from build123d import *

# Parameters (mm, degrees)
PAD_DEPTH       = 30
SKETCH004_R     = 9.7
POCKET_DEPTH    = 29
SKETCH005_R     = 9.7
POCKET001_DEPTH = 29
SKETCH006_R     = 1.5
POCKET002_DEPTH = 10
SKETCH007_R     = 1.5
POCKET003_DEPTH = 10
PAD001_DEPTH    = 10
SKETCH008_R     = 2.1
POCKET004_DEPTH = 7
SKETCH009_R     = 3.6
POCKET005_DEPTH = 2
FILLET_R        = 5


with BuildPart() as pocket003:
    # Sketch → Pad (new body, symmetric)
    with BuildSketch(Plane.XY):
        with BuildLine():
            ThreePointArc((-5.656854, 5.656854), (0, -8), (5.656854, 5.656854))
            Line((10.606602, 10.606602), (5.656854, 5.656854))
            ThreePointArc((0, -15), (13.858193, -5.740251), (10.606602, 10.606602))
            Line((-4.3e-05, -15), (0, -15))
            ThreePointArc((-15, -4.3e-05), (-10.606602, -10.606602), (-4.3e-05, -15))
            Line((-15, 0), (-15, -4.3e-05))
            ThreePointArc((-10.606602, 10.606602), (-13.858193, 5.740251), (-15, 0))
            Line((-5.656854, 5.656854), (-10.606602, 10.606602))
        make_face()
    extrude(amount=PAD_DEPTH, both=True)

    # Sketch004 → Pocket (cut)
    with BuildSketch(Plane.XY.offset(30)):
        Circle(SKETCH004_R)
    extrude(amount=-POCKET_DEPTH, mode=Mode.SUBTRACT)

    # Sketch005 → Pocket001 (cut)
    with BuildSketch(Plane(origin=(0, 0, -30), x_dir=(1, 0, 0), z_dir=(0, 0, -1))):
        Circle(SKETCH005_R)
    extrude(amount=-POCKET001_DEPTH, mode=Mode.SUBTRACT)

    # Sketch006 → Pocket002 (cut)
    with BuildSketch(Plane.XY.offset(30)):
        with Locations((-8, -8.944272)):
            Circle(SKETCH006_R)
    extrude(amount=-POCKET002_DEPTH, mode=Mode.SUBTRACT)

    # Sketch007 → Pocket003 (cut)
    with BuildSketch(Plane(origin=(0, 0, -30), x_dir=(1, 0, 0), z_dir=(0, 0, -1))):
        with Locations((-8, 8.944272)):
            Circle(SKETCH007_R)
    extrude(amount=-POCKET003_DEPTH, mode=Mode.SUBTRACT)


with BuildPart() as fusion:
    # Sketch003 → Pad001 (new body, symmetric)
    with BuildSketch(Plane.XY):
        with BuildLine():
            ThreePointArc((-13, 0), (0, -13), (13, 0))
            Line((13, 0), (13, -8))
            Line((13, -8), (25, -8))
            Line((25, -15), (25, -8))
            Line((-25, -15), (25, -15))
            Line((-25, -8), (-25, -15))
            Line((-13, -8), (-25, -8))
            Line((-13, 0), (-13, -8))
        make_face()
    extrude(amount=PAD001_DEPTH, both=True)

    # Sketch008 → Pocket004 (cut)
    with BuildSketch(Plane.XZ.offset(15)):
        with Locations((-19, 0)):
            Circle(SKETCH008_R)
        with Locations((19, 0)):
            Circle(SKETCH008_R)
    extrude(amount=-POCKET004_DEPTH, mode=Mode.SUBTRACT)

    # Sketch009 → Pocket005 (cut)
    with BuildSketch(Plane(origin=(0, -8, 0), x_dir=(-1, 0, 0), z_dir=(0, 1, 0))):
        with Locations((-19, 0)):
            Circle(SKETCH009_R)
        with Locations((19, 0)):
            Circle(SKETCH009_R)
    extrude(amount=-POCKET005_DEPTH, mode=Mode.SUBTRACT)

    # Fillet
    fillet_edges = [fusion.edges().sort_by_distance(p)[0] for p in [
        (25, -11.5, 10),
        (25, -11.5, -10),
        (-25, -11.5, 10),
        (-25, -11.5, -10),
    ]]
    fillet(fillet_edges, radius=FILLET_R)

    # Fusion: union Pocket003
    add(pocket003.part)


solid = fusion.part
Source: CAD feature listing. Evaluate the final solid. Frame: model axes, mm. A direction names the side the tool comes from. Give positions to 0.01 mm unless a question says otherwise; leave off trailing zeros. Write each loop counter-clockwise with the first axis right and the second up, starting at its lowest first coordinate (ties: lowest second). Pieces come first, ordered by that corner, then holes. Notation, with made-up numbers: (39.25, 30) - (91.25, 30) arc R24 ccw to (91.25, 45) - close; hole circle Ø4 at (-15, 33). An arc over 180 degrees is marked (long way). Write item = value, one per line. Start each with the question number.
Q1. Cut plane B-B, the plane y = 2. Return loops of the section in (x, z), then the cut area to 3 significant figures.
Q2. Material intervals for probe 1 along Z at (x, y) = (-19, -13.7); probe 2 along Z at (x, y) = (-19, -9); probe 3 along X at (y, z) = (-7.25, 22.5), sorted ascending.
Q3. Reachability of faces 1 (the cylindrical face through (-13.663, -6.189, 0.42)), 2 (the flat face through (15, -12, -10)), 3 (the cylindrical face through (-15.403, -8.986, 0.158)) from +Z, -Z, +X, -X, +Y, -Y: full face, straight path, thin tool, end or side. Return the list, or none.
Q4. Cut plane A-A, the plane x = 19. Return loops of the section in (y, z).
Q5. Pin query (flat end, axial travel): pin 1 Ø2.5 at (x, y) = (13, -10) entering from +Z; pin 2 Ø3 at (x, y) = (6, 0) entering from +Z; pin 3 Ø3.5 at (x, z) = (20.5, 1.5) entering from +Y; pin 4 Ø9.5 at (x, z) = (17.5, -3) entering from +Y. Return the tip coordinate at first contact, or that it passes through.
Q6. Cut plane D-D, the plane x = 4.5. Return loops of the section in (y, z), then the cut area to 3 significant figures.
Q7. Draft query along Z for faces 4 (the cylindrical face through (-16.997, -12.535, 0.631)), 5 (the flat face through (-15, -8, 0)), 6 (the flat face through (-8, -9, -20)), 7 (the cylindrical face through (22.597, -8.986, 0.158)). Return one class per face: +Z half, -Z half, draft (parallel to the pull), parting line (faces both ways), or undercut.
Computed values:
q1.outline = (-14.87, -30) - (-9.49, -30) - (-9.49, -1) - (-7.75, -1) - (-7.75, 1) - (-9.49, 1) - (-9.49, 30) - (-14.87, 30) - close; (7.75, -1) - (9.49, -1) - (9.49, -30) - (14.87, -30) - (14.87, 30) - (9.49, 30) - (9.49, 1) - (7.75, 1) - close
q1.area = 652 mm²
q2.probe_1 = -10 to -2.1, 2.1 to 10
q2.probe_2 = -10 to -3.6, 3.6 to 10
q2.probe_3 = -13.13 to -6.44, 6.44 to 13.13
q3.face_1 = -X
q3.face_2 = -Z, +X, -Y
q3.face_3 = +Y
q4.outline = (-15, -10) - (-8, -10) - (-8, -3.6) - (-10, -3.6) - (-10, -2.1) - (-15, -2.1) - close; (-15, 2.1) - (-10, 2.1) - (-10, 3.6) - (-8, 3.6) - (-8, 10) - (-15, 10) - close
q5.pin_1 = 10
q5.pin_2 = through
q5.pin_3 = -8
q5.pin_4 = 7.9
q6.outline = (-15, -10) - (-14.31, -10) - (-14.31, -30) - (-8.59, -30) - (-8.59, -1) - (-6.61, -1) - (-6.61, 1) - (-8.59, 1) - (-8.59, 30) - (-14.31, 30) - (-14.31, 10) - (-15, 10) - close
q6.area = 361 mm²
q7.face_4 = undercut
q7.face_5 = draft
q7.face_6 = -Z half
q7.face_7 = undercut
